Geometry check sheet. Reference: the model listing, model coordinates, mm. A direction names the side the tool comes from. Give positions to 0.01 mm unless a question says otherwise; leave off trailing zeros. Loops run counter-clockwise (first coordinate to the right, second up) from the corner with the lowest first, then second, coordinate; pieces in that order, holes last. Notation, with made-up numbers: (37, 50.5) -> (48, 50.5) arc R7 ccw to (48, 57.5) -> close; hole circle Ø11 at (88, 69). An arc over 180 degrees is marked (long way). Write item = value, one per line.
```python
from build123d import *

# Parameters (mm, degrees)
SKETCH1_W           = 38
SKETCH1_H           = 120
BOSS_EXTRUDE1_DEPTH = 15
SKETCH2_W           = 21
SKETCH2_H           = 41
CUT_EXTRUDE2_DEPTH  = 15
SKETCH3_R           = 1.75
CUT_EXTRUDE4_DEPTH  = 15
SKETCH6_W           = 12.0625825
SKETCH6_H           = 31
CUT_EXTRUDE8_DEPTH  = 38
SKETCH8_R           = 7.155544399
SKETCH8_R_2         = 1
CUT_EXTRUDE10_DEPTH = 10
FILLET2_R           = 10
FILLET3_R           = 10


with BuildPart() as part:
    # Sketch1 → Boss-Extrude1 (new body)
    with BuildSketch(Plane.XY):
        with Locations((-1.743801653, -11.107438017)):
            Rectangle(SKETCH1_W, SKETCH1_H)
    extrude(amount=BOSS_EXTRUDE1_DEPTH)

    # Sketch2 → Cut-Extrude2 (cut)
    with BuildSketch(Plane.XY.offset(15)):
        with Locations((-1.743801653, -35.607438017)):
            Rectangle(SKETCH2_W, SKETCH2_H)
    extrude(amount=-CUT_EXTRUDE2_DEPTH, mode=Mode.SUBTRACT)

    # Sketch3 → Cut-Extrude4 (cut)
    with BuildSketch(Plane.XY.offset(15)):
        with Locations((-6.243801653, -9.517630565)):
            Circle(SKETCH3_R)
        with Locations((3.756198347, -9.517630565)):
            Circle(SKETCH3_R)
        with Locations((-6.243801653, -62.215563881)):
            Circle(SKETCH3_R)
        with Locations((3.756198347, -62.215563881)):
            Circle(SKETCH3_R)
    extrude(amount=-CUT_EXTRUDE4_DEPTH, mode=Mode.SUBTRACT)

    # Sketch6 → Cut-Extrude8 (cut)
    with BuildSketch(Plane(origin=(17.256198347, 0, 0), x_dir=(0, 0, -1), z_dir=(1, 0, 0))):
        with Locations((-7.5, 28.392561983)):
            Rectangle(SKETCH6_W, SKETCH6_H)
    extrude(amount=-CUT_EXTRUDE8_DEPTH, mode=Mode.SUBTRACT)

    # Sketch8 → Cut-Extrude10 (cut)
    with BuildSketch(Plane(origin=(0, 48.892561983, 0), x_dir=(1, 0, 0), z_dir=(0, 1, 0))):
        with Locations(Location((-10.864699175, -7.628809465, 0), (0, 0, 270))):
            Circle(SKETCH8_R)
        with Locations(Location((-19.364699175, -7.340375333, 0), (0, 0, 270))):
            Circle(SKETCH8_R_2)
        with Locations(Location((-2.364699175, -7.628809465, 0), (0, 0, 270))):
            Circle(SKETCH8_R_2)
    extrude(amount=-CUT_EXTRUDE10_DEPTH, mode=Mode.SUBTRACT)

    # Fillet2
    # the kernel refuses this fillet: 10 mm, written as the material it takes off along each edge
    with BuildSketch(Plane(origin=(-20.743801653, -96.107438017, 15), x_dir=(0, 0, -1), z_dir=(0, 1, 0))) as fillet2_piece_1:
        with BuildLine():
            CenterArc((FILLET2_R, -FILLET2_R), FILLET2_R, 90, 90)
            Line((0, -FILLET2_R), (0, 0))
            Line((0, 0), (FILLET2_R, 0))
        make_face()
    extrude(amount=170, mode=Mode.SUBTRACT)
    with BuildSketch(Plane(origin=(17.256198347, 73.892561983, 15), x_dir=(-1, 0, 0), z_dir=(0, -1, 0))) as fillet2_piece_2:
        with BuildLine():
            CenterArc((FILLET2_R, FILLET2_R), FILLET2_R, 180, 90)
            Line((0, FILLET2_R), (0, 0))
            Line((0, 0), (FILLET2_R, 0))
        make_face()
    extrude(amount=170, mode=Mode.SUBTRACT)

    # Fillet3
    # the kernel refuses this fillet: 10 mm, written as the material it takes off along each edge
    with BuildSketch(Plane(origin=(-20.743801653, -92.758073111, 0), x_dir=(1, 0, 0), z_dir=(0, 1, 0)), Plane(origin=(17.256198347, 70.543197078, 0), x_dir=(-1, 0, 0), z_dir=(0, -1, 0))) as fillet3_piece_1:
        with BuildLine():
            CenterArc((8.660254038, -10), FILLET3_R, 90, 60)
            Line((0, -5), (-0.173205081, -4.9))
            ThreePointArc((-0.173205081, -4.9), (-0.2, -2.5), (-0.2, 0))
            Line((-0.2, 0), (0, 0.2))
            Line((0, 0.2), (8.660254038, 0.2))
            Line((8.660254038, 0.2), (8.660254038, 0))
        make_face()
    extrude(amount=163.301270189, mode=Mode.SUBTRACT)


solid = part.part
```
Item 1: Section check A-A, the plane x = 0. Record the cut outline in (y, z), plus the area to 3 significant figures.
Answer:
outline = (-71.11, 0) -> (-56.11, 0) -> (-56.11, 15) -> (-71.11, 15) -> close; (-15.11, 0) -> (48.89, 0) -> (48.89, 15) -> (-15.11, 15) -> close; hole (12.89, 1.47) -> (43.89, 1.47) -> (43.89, 13.53) -> (12.89, 13.53) -> close
area = 811 mm^2
Item 2: Section check B-B, the plane y = 20. Record the cut outline in (x, z), plus the area to 3 significant figures.
Answer:
outline = (-17.3, 1.47) arc R10 ccw to (-12.08, 0) -> (8.6, 0) arc R10 ccw to (13.81, 1.47) -> close; (-15.96, 13.53) -> (12.47, 13.53) arc R10 ccw to (7.26, 15) -> (-10.74, 15) arc R10 ccw to start
area = 77.6 mm^2
Item 3: Thickness scan on L1, parallel to Z at x = -11, y = 19; L2, parallel to Y at x = -6.5, z = 0.5; L3, parallel to X at y = -16, z = 5. Record the ranges inside material, lowest first. Write a range as [from, to].
Answer:
L1 = [0, 1.47], [13.53, 15]
L2 = [-71.11, -63.95], [-60.48, -56.11], [-15.11, -11.25], [-7.79, 48.89]
L3 = [-20.74, -12.24], [8.76, 17.26]
Item 4: Draft check along X on faces 1 (the cylindrical face through (3.377, -63.924, 7.605)), 2 (the cylindrical face through (-17.02, -25.281, 1.303)), 3 (the flat face through (-2, 28, 1.469)), 4 (the cylindrical face through (13.53, -23.6, 1.3)). Enter one of: +X half, -X half, draft (parallel to the pull), parting line (faces both ways), or undercut.
Answer:
face_1 = undercut
face_2 = -X half
face_3 = draft
face_4 = +X half
Item 5: Section check C-C, the plane z = 3.75. Record the cut outline in (x, y).
Answer:
outline = (-19.89, -71.11) -> (16.4, -71.11) -> (16.4, 12.89) -> (-19.89, 12.89) -> close; (-19.89, 43.89) -> (-16.88, 43.89) -> (-16.88, 48.89) -> (-19.89, 48.89) -> close; (-4.85, 43.89) -> (16.4, 43.89) -> (16.4, 48.89) -> (-4.85, 48.89) -> close; hole (-12.24, -56.11) -> (8.76, -56.11) -> (8.76, -15.11) -> (-12.24, -15.11) -> close; hole circle Ø3.5 at (-6.24, -62.22); hole circle Ø3.5 at (-6.24, -9.52); hole circle Ø3.5 at (3.76, -62.22); hole circle Ø3.5 at (3.76, -9.52)
Item 6: Tool access check on faces 5 (the flat face through (-2, -56.107, 8)), 6 (the flat face through (5, 43.893, 8)), 7 (the cylindrical face through (-13.605, 45.074, 14.239)). Record the directions out of +Z, -Z, +X, -X, +Y, -Y that give a thin tool (end or side, any length) a straight path to the whole face; none if there is none.
Answer:
face_5 = +Z, -Z
face_6 = +X, -X
face_7 = +Y
Item 7: Gauge pin test, flat ends, axial feed: pin 1 (0.5 mm diameter, centred on x = -12.5, z = 1, fed in from +Y); pin 2 (1 mm diameter, centred on x = 10.5, y = -48.5, fed in from -Z); pin 3 (1.6 mm diameter, centred on x = -19.36, z = 7.34, fed in from +Y). Record the tip position at first contact, or that the pin passes through.
Answer:
pin_1 = 38.89
pin_2 = 0.1
pin_3 = 12.89
Item 8: Section check D-D, the plane y = -1. Record the cut outline in (x, z).
Answer:
outline = (-20.74, 5) arc R10 ccw to (-12.08, 0) -> (8.6, 0) arc R10 ccw to (17.26, 5) arc R10 ccw to (7.26, 15) -> (-10.74, 15) arc R10 ccw to start
